The model under review builds one solid part; all positions refer to its coordinate system, in mm. Face numbers are marked on the shaded views. A direction names the side the tool comes from. Round coordinates to 2 decimals unless told otherwise and drop trailing zeros. Write each loop counter-clockwise with the first axis right and the second up, starting at its lowest first coordinate (ties: lowest second). Pieces come first, ordered by that corner, then holes. Notation, with made-up numbers: (59.5, -37.75) -> (86.5, -37.75) arc R8 cw to (86.5, -33.75) -> close; hole circle Ø5 at (-5.75, -30.75). An arc over 180 degrees is marked (long way). Answer in a Markdown table with one row per item. Add a question column.
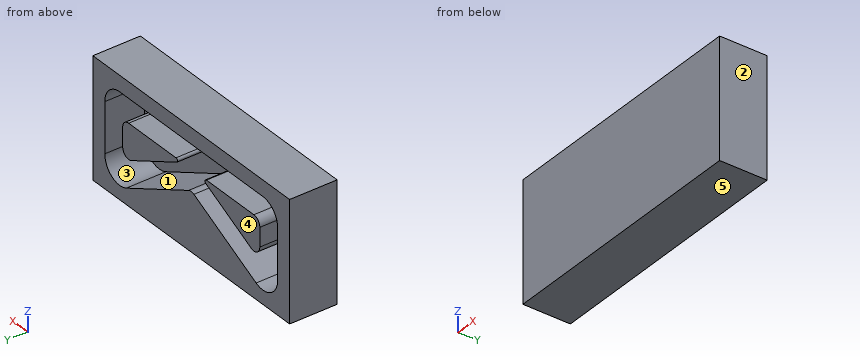
```python
from build123d import *

# Parameters (mm, degrees)
BOSS_EXTRUDE1_DEPTH   = 5
BOSS_EXTRUDE1_2_DEPTH = 5
SKETCH1_W             = 33
SKETCH1_H             = 15.045084972
BOSS_EXTRUDE1_3_DEPTH = 5
SKETCH2_W             = 33
SKETCH2_H             = 15.045084972
BOSS_EXTRUDE3_DEPTH   = 1


with BuildPart() as part:
    # Sketch1 → Boss-Extrude1 (new body)
    with BuildSketch(Plane(origin=(0, 0, 0), x_dir=(1, 0, 0), z_dir=(0, 1, 0))):
        with BuildLine():
            Line((-0.947213595, 0.473606798), (-8.552786405, 4.276393202))
            ThreePointArc((-8.552786405, 4.276393202), (-9.525731112, 4.23261682), (-10, 3.381966011))
            Line((-10, 3.381966011), (-10, 1))
            ThreePointArc((-10, 1), (-9.707106781, 0.292893219), (-9, 0))
            Line((-9, 0), (-1.059016994, 0))
            ThreePointArc((-1.059016994, 0), (-0.815704747, 0.19256177), (-0.947213595, 0.473606798))
        make_face()
    extrude(amount=BOSS_EXTRUDE1_DEPTH)



with BuildPart() as body_2:
    # Sketch1 → Boss-Extrude1 2 (new body)
    with BuildSketch(Plane(origin=(0, 0, 0), x_dir=(1, 0, 0), z_dir=(0, 1, 0))):
        with BuildLine():
            Line((12, 0), (4.059016994, 0))
            ThreePointArc((4.059016994, 0), (3.815704747, 0.19256177), (3.947213595, 0.473606798))
            Line((3.947213595, 0.473606798), (11.552786405, 4.276393202))
            ThreePointArc((11.552786405, 4.276393202), (12.525731112, 4.23261682), (13, 3.381966011))
            Line((13, 3.381966011), (13, 1))
            ThreePointArc((13, 1), (12.707106781, 0.292893219), (12, 0))
        make_face()
    extrude(amount=BOSS_EXTRUDE1_2_DEPTH)


with BuildPart() as body_3:
    # Sketch1 → Boss-Extrude1 3 (new body)
    with BuildSketch(Plane(origin=(0, 0, 0), x_dir=(1, 0, 0), z_dir=(0, 1, 0))):
        with Locations((1.5, 2.522542486)):
            Rectangle(SKETCH1_W, SKETCH1_H)
        with BuildLine():
            Line((1.052786405, 2.827708764), (-9.381966011, 8.045084972))
            ThreePointArc((-9.381966011, 8.045084972), (-11.81432778, 7.935644015), (-13, 5.809016994))
            Line((-13, 5.809016994), (-13, -0.5))
            ThreePointArc((-13, -0.5), (-12.267766953, -2.267766953), (-10.5, -3))
            Line((-10.5, -3), (13.5, -3))
            ThreePointArc((13.5, -3), (15.267766953, -2.267766953), (16, -0.5))
            Line((16, -0.5), (16, 5.809016994))
            ThreePointArc((16, 5.809016994), (14.81432778, 7.935644015), (12.381966011, 8.045084972))
            Line((12.381966011, 8.045084972), (1.947213595, 2.827708764))
            ThreePointArc((1.947213595, 2.827708764), (1.5, 2.722135955), (1.052786405, 2.827708764))
        make_face(mode=Mode.SUBTRACT)
    extrude(amount=BOSS_EXTRUDE1_3_DEPTH)


with BuildPart() as part_1:
    add(part.part)

    add(body_2.part)  # Boss-Extrude3 merges body 2

    add(body_3.part)  # Boss-Extrude3 merges body 3
    # Sketch2 → Boss-Extrude3 (add)
    with BuildSketch(Plane.XZ):
        with Locations((1.5, -2.522542486)):
            Rectangle(SKETCH2_W, SKETCH2_H)
    extrude(amount=BOSS_EXTRUDE3_DEPTH)


solid = part_1.part
```
1. Add section C-C on x = 1.5. Write out the cut boundary in (y, z), plus the area to 3 significant figures.
2. Add section A-A on y = 0.5. Write out the cut boundary in (x, z).
3. Add section B-B on z = -2. Write out the cut boundary in (x, y).
4. Tool access review of the marked faces 1 and 2: name each direction out of +Z, -Z, +X, -X, +Y, -Y from which nothing blocks a thin tool from reaching the whole face with its end or side.
5. Add section D-D on z = -5.5. Write out the cut boundary in (x, y).
6. For L1, parallel to Z at x = -7, y = 1.25; L2, parallel to Z at x = 9, y = 1.55; L3, parallel to X at y = 4.7, z = -3.75, list the stretches that pass through material, from the lowest coordinate up.
7. Mouldability with a two-part tool opening along Z and no side actions: class the marked faces 3, 4 and 5 as pulls with the +Z half, pulls with the -Z half, needs draft (parallel to the pull), parting line crosses it, or undercut.
Filled in:
| question | item | result |
|---|---|---|
| 1 | outline | (-1, -10.05) -> (5, -10.05) -> (5, -2.72) -> (0, -2.72) -> (0, 3) -> (5, 3) -> (5, 5) -> (-1, 5) -> close |
| 1 | area | 61.7 mm² |
| 2 | outline | (-15, -10.05) -> (18, -10.05) -> (18, 5) -> (-15, 5) -> close; (-10, -3.38) arc R1 ccw to (-8.55, -4.28) -> (-0.95, -0.47) arc R0.25 ccw to (-1.06, 0) -> (-9, 0) arc R1 ccw to (-10, -1) -> close; (3.95, -0.47) -> (11.55, -4.28) arc R1 ccw to (13, -3.38) -> (13, -1) arc R1 ccw to (12, 0) -> (4.06, 0) arc R0.25 ccw to start; hole (-13, -5.81) arc R2.5 ccw to (-9.38, -8.05) -> (1.05, -2.83) arc R1 cw to (1.95, -2.83) -> (12.38, -8.05) arc R2.5 ccw to (16, -5.81) -> (16, 0.5) arc R2.5 ccw to (13.5, 3) -> (-10.5, 3) arc R2.5 ccw to (-13, 0.5) -> close |
| 3 | outline | (-15, -1) -> (18, -1) -> (18, 5) -> (16, 5) -> (16, 0) -> (13, 0) -> (13, 5) -> (7, 5) -> (7, 0) -> (-4, 0) -> (-4, 5) -> (-10, 5) -> (-10, 0) -> (-13, 0) -> (-13, 5) -> (-15, 5) -> close |
| 4 | face 1 | +Y |
| 4 | face 2 | +Z, -Z, +X, +Y, -Y |
| 5 | outline | (-15, -1) -> (18, -1) -> (18, 5) -> (16, 5) -> (16, 0) -> (7.29, 0) -> (7.29, 5) -> (-4.29, 5) -> (-4.29, 0) -> (-13, 0) -> (-13, 5) -> (-15, 5) -> close |
| 6 | L1 | -10.05 to -6.85, -3.5 to 0, 3 to 5 |
| 6 | L2 | -10.05 to -6.35, -3 to 0, 3 to 5 |
| 6 | L3 | -15 to -13, -9.93 to -7.5, -0.79 to 3.79, 10.5 to 12.93, 16 to 18 |
| 7 | face 3 | undercut |
| 7 | face 4 | needs draft |
| 7 | face 5 | pulls with the -Z half |
